Part model, mm, in its own coordinate system. Face numbers are marked on the shaded views. Round coordinates to 2 decimals unless told otherwise and drop trailing zeros. Order: outer loops, then holes, each group sorted by start corner. A loop starts at its lowest first (then second) coordinate and runs counter-clockwise, first axis right, second up. Notation, with made-up numbers: (21.25, 7) - (42.25, 7) arc R19 cw to (42.25, 11) - close; hole circle Ø3 at (67, 53.25). An arc over 180 degrees is marked (long way). Answer as a JSON object with one key per item and string values.
```python
from build123d import *

# Parameters (mm, degrees)
SKETCH1_W           = 233.09940225
SKETCH1_H           = 18.807132604
SKETCH1_R           = 3.7970867
BOSS_EXTRUDE1_DEPTH = 50
SKETCH3_R           = 4.00110176
BOSS_EXTRUDE2_DEPTH = 10
BOSS_EXTRUDE5_START = -233
SKETCH3_2_R         = 4.00110176
BOSS_EXTRUDE5_DEPTH = 10
SKETCH4_R           = 4.00110176
BOSS_EXTRUDE6_DEPTH = 233
CUT_EXTRUDE1_REACH  = 52.07
SKETCH5_W           = 194.621538706
SKETCH5_H           = 28.304823728


with BuildPart() as part:
    # Sketch1 → Boss-Extrude1 (new body)
    with BuildSketch(Plane.XY):
        with Locations((87.483442541, -10.016557459)):
            Rectangle(SKETCH1_W, SKETCH1_H)
        with Locations((-10.016557459, -10.016557459)):
            Circle(SKETCH1_R, mode=Mode.SUBTRACT)
        with Locations((184.983442541, -10.016557459)):
            Circle(SKETCH1_R, mode=Mode.SUBTRACT)
    extrude(amount=BOSS_EXTRUDE1_DEPTH)

    # Sketch3 → Boss-Extrude2 (add)
    with BuildSketch(Plane.ZY.offset(29.066258584)):
        with BuildLine():
            Line((10.743495107, -0.612991157), (10.743495107, 16.393198277))
            ThreePointArc((10.743495107, 16.393198277), (25, 30.64970317), (39.256504893, 16.393198277))
            Line((39.256504893, 16.393198277), (39.256504893, -0.612991157))
            Line((39.256504893, -0.612991157), (10.743495107, -0.612991157))
        make_face()
        with Locations((25, 16.393198277)):
            Circle(SKETCH3_R, mode=Mode.SUBTRACT)
    extrude(amount=-BOSS_EXTRUDE2_DEPTH)

    # Sketch3_2 → Boss-Extrude5 (add)
    with BuildSketch(Plane.ZY.offset(29.066258584).offset(BOSS_EXTRUDE5_START)):
        with BuildLine():
            Line((10.743495107, -0.612991157), (10.743495107, 16.393198277))
            ThreePointArc((10.743495107, 16.393198277), (25, 30.64970317), (39.256504893, 16.393198277))
            Line((39.256504893, 16.393198277), (39.256504893, -0.612991157))
            Line((39.256504893, -0.612991157), (10.743495107, -0.612991157))
        make_face()
        with Locations((25, 16.393198277)):
            Circle(SKETCH3_2_R, mode=Mode.SUBTRACT)
    extrude(amount=BOSS_EXTRUDE5_DEPTH)

    # Sketch4 → Boss-Extrude6 (add)
    with BuildSketch(Plane(origin=(203.933741416, 0, 0), x_dir=(0, 0, -1), z_dir=(1, 0, 0))):
        with Locations((-25, 16.393198277)):
            Circle(SKETCH4_R)
    extrude(amount=-BOSS_EXTRUDE6_DEPTH)

    # Sketch5 → Cut-Extrude1 (cut, up to next)
    with BuildSketch(Plane.XZ.offset(19.420123761), mode=Mode.PRIVATE) as cut_extrude1_sk1:
        with Locations((87.483442541, 25)):
            Rectangle(SKETCH5_W, SKETCH5_H)
    cut_extrude1_tool1 = extrude(cut_extrude1_sk1.sketch, amount=-CUT_EXTRUDE1_REACH, mode=Mode.PRIVATE) & part.part
    add(cut_extrude1_tool1.solids().sort_by_distance((87.483443, -19.420124, 25))[0], mode=Mode.SUBTRACT)


solid = part.part
```
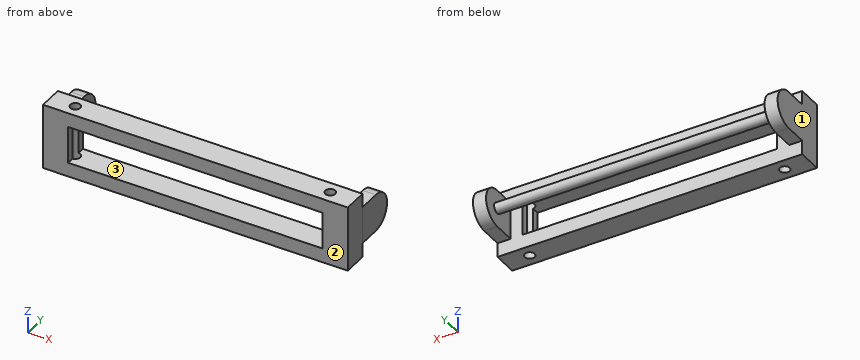
Item 1: Probe L1, parallel to X at y = -14.5, z = 21.5; L2, parallel to X at y = 15, z = 11; L3, parallel to Z at x = 5, y = -7. List the from-to ranges inside material, lowest first. Write a range as from..to.
Taken from the geometry:
{"L1": "-29.07..-9.83, 184.79..204.03", "L2": "-29.07..-19.07, 193.93..203.93", "L3": "0..10.85, 39.15..50"}
Item 2: Cut at B-B (y = 5). Write the cut outline in (x, z), plus the area to 3 significant figures.
Taken from the geometry:
{"outline": "(-29.07, 10.74) - (-19.07, 10.74) - (-19.07, 39.26) - (-29.07, 39.26) - close; (193.93, 10.74) - (203.93, 10.74) - (203.93, 39.26) - (193.93, 39.26) - close", "area": "570 mm2"}
Item 3: Cut at A-A (x = 69.5). Write the cut outline in (y, z).
Taken from the geometry:
{"outline": "(-19.42, 0) - (-0.61, 0) - (-0.61, 10.85) - (-19.42, 10.85) - close; (-19.42, 39.15) - (-0.61, 39.15) - (-0.61, 50) - (-19.42, 50) - close; circle Ø8 at (16.39, 25)"}
Item 4: Cut at C-C (z = 37). Write the cut outline in (x, y), plus the area to 3 significant figures.
Taken from the geometry:
{"outline": "(-29.07, -19.42) - (-9.83, -19.42) - (-9.83, -13.81) arc R3.8 cw (long way) to (-9.83, -6.22) - (-9.83, -0.61) - (-19.07, -0.61) - (-19.07, 24.09) - (-29.07, 24.09) - close; (184.79, -19.42) - (204.03, -19.42) - (204.03, -0.61) - (203.93, -0.61) - (203.93, 24.09) - (193.93, 24.09) - (193.93, -0.61) - (184.79, -0.61) - (184.79, -6.22) arc R3.8 cw (long way) to (184.79, -13.81) - close", "area": "1,170 mm2"}
Item 5: Drop flat-ended pins along their axis: P1, Ø3, axis at x = -22.5, y = 9, coming from the -Z side; P2, Ø1.5, axis at x = 69.5, y = 15.5, coming from the -Z side; P3, Ø7, axis at x = -10.02, y = -10.02, coming from the +Z side; P4, Ø1, axis at x = 30.5, z = 26.5, coming from the +Y side. Give the stop position or say it passes through.
Taken from the geometry:
{"P1": "z = 10.74", "P2": "z = 21", "P3": "through", "P4": "y = 20.27"}
Item 6: Cut at D-D (z = 25). Write the cut outline in (x, y).
Taken from the geometry:
{"outline": "(-29.07, -19.42) - (-9.83, -19.42) - (-9.83, -13.81) arc R3.8 cw (long way) to (-9.83, -6.22) - (-9.83, -0.61) - (-19.07, -0.61) - (-19.07, 12.39) - (193.93, 12.39) - (193.93, -0.61) - (184.79, -0.61) - (184.79, -6.22) arc R3.8 cw (long way) to (184.79, -13.81) - (184.79, -19.42) - (204.03, -19.42) - (204.03, -0.61) - (203.93, -0.61) - (203.93, 30.65) - (193.93, 30.65) - (193.93, 20.39) - (-19.07, 20.39) - (-19.07, 30.65) - (-29.07, 30.65) - close"}
Item 7: Two-plate mould, pull along X, no slides. Class the marked faces 1, 2 and 3: pulls with the +X half, pulls with the -X half, needs draft (parallel to the pull), parting line crosses it, or undercut.
Taken from the geometry:
{"face 1": "pulls with the -X half", "face 2": "needs draft", "face 3": "undercut"}
